The model under review builds one solid part; all positions refer to its coordinate system, in mm. Face numbers are marked on the shaded views. A direction names the side the tool comes from. Coordinates: 2 decimals unless noted, no trailing zeros. Loops run counter-clockwise (first coordinate to the right, second up) from the corner with the lowest first, then second, coordinate; pieces in that order, holes last. Notation, with made-up numbers: (19.5, 20.25) - (33.5, 20.25) arc R25 ccw to (33.5, 32.25) - close; hole circle Ø2 at (-28.75, -22). An arc over 180 degrees is marked (long way). Answer in a Markdown table with one row per item. Add a question column.
(1) For P1, Ø3, axis at y = -14, z = -58.5, coming from the -X side; P2, Ø12.5, axis at y = -14.5, z = 54.5, coming from the +X side; P3, Ø9.5, axis at x = 172, y = -13, coming from the -Z side (3 decimals), all flat-tipped, find the tip position at first contact; note any pin that passes through.
(2) Machinability: for the marked faces 4 and 5, which of the approach directions +Z, -Z, +X, -X, +Y, -Y give a long, thin tool a straight path to every point of the face, cutting with its end or side? Answer none if there is none.
(3) For line 1 along Z through (x, y) = (20.5, -16.25); line 2 along X through (y, z) = (-16.75, 6.5); line 3 along Z through (x, y) = (-77, -9.25), list the stretches that pass through material, from the lowest coordinate up.
(4) Mouldability with a two-part tool opening along X and no side actions: class the marked faces 1, 2 and 3 as +X half, -X half, draft (parallel to the pull), parting line (faces both ways), or undercut.
(5) We need section C-C on x = -123.5. Write out the cut boundary in (y, z).
(6) We need section B-B on z = 1. Write out the cut boundary in (x, y), plus the area to 3 significant figures.
(7) We need section A-A on x = -37. Write out the cut boundary in (y, z).
(8) We need section D-D on y = -4. Give the number of separate pieces and of enclosed holes in the cut face, plus the area to 3 significant figures.
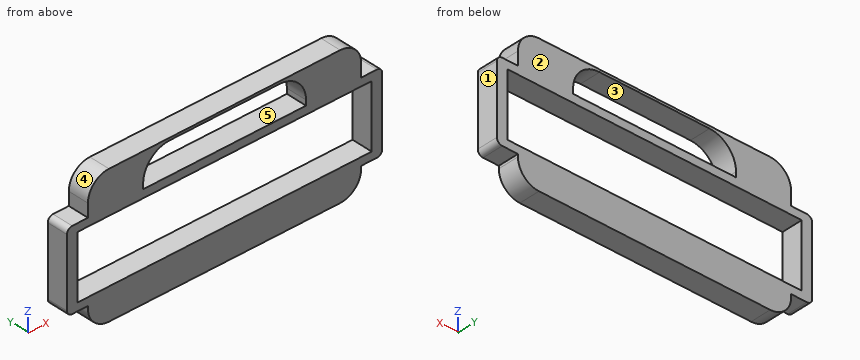
from build123d import *

# Parameters (mm, degrees)
F0_W     = 330.2
F0_H     = 41.275
F0_H_2   = 9.525
F0_H_3   = 28.575
F1_DEPTH = 25.4
F2_R     = 25.4
F3_R     = 6.35


with BuildPart() as f1:
    # F0 (on Front) → F1 (new body)
    with BuildSketch(Plane.XZ):
        with Locations((0, 68.2625)):
            Rectangle(F0_W, F0_H)
        Polygon((66.4316704035, 85.9683295965), (98.425, 85.9683295965), (98.425, 53.975), (98.425, 47.8683295965), (-98.425, 47.8683295965), (-98.425, 53.975), (-98.425, 85.9683295965), (-66.4316704035, 85.9683295965), align=None, mode=Mode.SUBTRACT)
        with BuildLine():
            ThreePointArc((-98.425, 53.975), (-89.0543707139, 76.5977003104), (-66.4316704035, 85.9683295965))
            Line((-66.4316704035, 85.9683295965), (-98.425, 85.9683295965))
            Line((-98.425, 85.9683295965), (-98.425, 53.975))
        make_face()
        with BuildLine():
            Line((98.425, 53.975), (98.425, 85.9683295965))
            Line((98.425, 85.9683295965), (66.4316704035, 85.9683295965))
            ThreePointArc((66.4316704035, 85.9683295965), (89.0543707139, 76.5977003104), (98.425, 53.975))
        make_face()
        Polygon((-190.5, -47.625), (-165.1, -47.625), (-165.1, -38.1), (-177.8, -38.1), (-177.8, 38.1), (-165.1, 38.1), (-165.1, 47.625), (-190.5, 47.625), align=None)
        with Locations((0, 42.8625)):
            Rectangle(F0_W, F0_H_2)
        Polygon((165.1, -47.625), (190.5, -47.625), (190.5, 47.625), (165.1, 47.625), (165.1, 38.1), (177.8, 38.1), (177.8, -38.1), (165.1, -38.1), align=None)
        with Locations((0, -42.8625)):
            Rectangle(F0_W, F0_H_2)
        with Locations((0, -61.9125)):
            Rectangle(F0_W, F0_H_3)
    extrude(amount=F1_DEPTH)

    # F2
    f2_edges = [f1.edges().sort_by_distance(p)[0] for p in [
        (-165.1, -12.7, 88.9),
        (165.1, -12.7, 88.9),
        (-165.1, -12.7, -76.2),
        (165.1, -12.7, -76.2),
    ]]
    fillet(f2_edges, radius=F2_R)

    # F3
    f3_edges = [f1.edges().sort_by_distance(p)[0] for p in [
        (-190.5, -12.7, 47.625),
        (-190.5, -12.7, -47.625),
        (190.5, -12.7, -47.625),
        (190.5, -12.7, 47.625),
    ]]
    fillet(f3_edges, radius=F3_R)


solid = f1.part
Outcome:
| question | item | result |
|---|---|---|
| 1 | P1 | x = -164.33 |
| 1 | P2 | x = 165.1 |
| 1 | P3 | z = -47.625 |
| 2 | face 4 | +Z, -X, +Y, -Y |
| 2 | face 5 | +Y, -Y |
| 3 | line 1 | -76.2 to -38.1, 38.1 to 47.87, 85.97 to 88.9 |
| 3 | line 2 | -190.5 to -177.8, 177.8 to 190.5 |
| 3 | line 3 | -76.2 to -38.1, 38.1 to 47.87, 84.17 to 88.9 |
| 4 | face 1 | +X half |
| 4 | face 2 | draft |
| 4 | face 3 | undercut |
| 5 | outline | (-25.4, -76.2) - (0, -76.2) - (0, -38.1) - (-25.4, -38.1) - close; (-25.4, 38.1) - (0, 38.1) - (0, 88.9) - (-25.4, 88.9) - close |
| 6 | outline | (-190.5, -25.4) - (-177.8, -25.4) - (-177.8, 0) - (-190.5, 0) - close; (177.8, -25.4) - (190.5, -25.4) - (190.5, 0) - (177.8, 0) - close |
| 6 | area | 645 mm² |
| 7 | outline | (-25.4, -76.2) - (0, -76.2) - (0, -38.1) - (-25.4, -38.1) - close; (-25.4, 38.1) - (0, 38.1) - (0, 47.87) - (-25.4, 47.87) - close; (-25.4, 85.97) - (0, 85.97) - (0, 88.9) - (-25.4, 88.9) - close |
| 8 | separate pieces | 1 |
| 8 | enclosed holes | 2 |
| 8 | area | 24,600 mm² |
